from build123d import *

# Parameters (mm, degrees)
SKETCH1_R             = 60.625
SKETCH1_R_2           = 45
BOSS_EXTRUDE1_DEPTH   = 4
SKETCH2_R             = 49
SKETCH2_R_2           = 45
BOSS_EXTRUDE2_DEPTH   = 50.5
SKETCH4_W             = 8
SKETCH4_H             = 40.5
BOSS_EXTRUDE4_DEPTH   = 7
SKETCH4_W_2           = 27
SKETCH4_H_2           = 10
BOSS_EXTRUDE4_2_DEPTH = 7
BOSS_EXTRUDE5_DEPTH   = 4
SKETCH6_R             = 5
CUT_EXTRUDE2_DEPTH    = 52
CUT_EXTRUDE6_DEPTH    = 100.503925853
SKETCH15_R            = 0.5
CUT_EXTRUDE7_DEPTH    = 4.5
SKETCH15_3_R          = 0.5
CUT_EXTRUDE8_DEPTH    = 4.5
BOSS_EXTRUDE6_DEPTH   = 6.75


with BuildPart() as part:
    # Sketch1 → Boss-Extrude1 (new body)
    with BuildSketch(Plane(origin=(0, 0, 0), x_dir=(1, 0, 0), z_dir=(0, 1, 0))):
        with Locations(Location((0, 0, 0), (0, 0, 270))):
            Circle(SKETCH1_R)
        with Locations(Location((0, 0, 0), (0, 0, 270))):
            Circle(SKETCH1_R_2, mode=Mode.SUBTRACT)
    extrude(amount=BOSS_EXTRUDE1_DEPTH)

    # Sketch2 → Boss-Extrude2 (add)
    with BuildSketch(Plane(origin=(0, 4, 0), x_dir=(1, 0, 0), z_dir=(0, 1, 0))):
        with Locations(Location((0, 0, 0), (0, 0, 270))):
            Circle(SKETCH2_R)
        with Locations(Location((0, 0, 0), (0, 0, 270))):
            Circle(SKETCH2_R_2, mode=Mode.SUBTRACT)
    extrude(amount=BOSS_EXTRUDE2_DEPTH)



with BuildPart() as body_2:
    # Sketch4 → Boss-Extrude4 (new, symmetric)
    with BuildSketch(Plane.XY):
        with Locations((10, 20.25)):
            Rectangle(SKETCH4_W, SKETCH4_H)
    extrude(amount=BOSS_EXTRUDE4_DEPTH, both=True)


with BuildPart() as body_3:
    # Sketch4 → Boss-Extrude4 2 (new, symmetric)
    with BuildSketch(Plane.XY):
        with Locations((-30.5, 35.5)):
            Rectangle(SKETCH4_W_2, SKETCH4_H_2)
    extrude(amount=BOSS_EXTRUDE4_2_DEPTH, both=True)

    # Sketch15<3> → Cut-Extrude8 (cut)
    with BuildSketch(Plane(origin=(0, 40.5, 0), x_dir=(1, 0, 0), z_dir=(0, 1, 0))):
        with Locations(Location((-19.5, 0, 0), (0, 0, 270))):
            Circle(SKETCH15_3_R)
        with Locations(Location((8.5, 0, 0), (0, 0, 270))):
            Circle(SKETCH15_3_R)
    extrude(amount=-CUT_EXTRUDE8_DEPTH, mode=Mode.SUBTRACT)


with BuildPart() as part_1:
    add(part.part)

    add(body_2.part)  # Boss-Extrude5 merges body 2
    # Sketch5 → Boss-Extrude5 (add)
    with BuildSketch(Plane(origin=(0, 0, 0.832419338), x_dir=(1, 0, 0), z_dir=(0, -1, 0))):
        with BuildLine():
            Line((0.92268666, 14.579552818), (36.10584122, 30.137929754))
            ThreePointArc((36.10584122, 30.137929754), (47.46850162, -1.287411864), (36.651216878, -32.904630242))
            Line((36.651216878, -32.904630242), (0.92268666, -16.029114558))
            Line((0.92268666, -16.029114558), (0.92268666, 14.579552818))
        make_face()
    extrude(amount=-BOSS_EXTRUDE5_DEPTH)

    # Sketch6 → Cut-Extrude2 (cut)
    with BuildSketch(Plane.XY):
        with Locations(Location((-11.847358964, 24.485616242, 0), (0, 0, 180))):
            Circle(SKETCH6_R)
    extrude(amount=CUT_EXTRUDE2_DEPTH, mode=Mode.SUBTRACT)

    # Sketch11 → Cut-Extrude6 (cut, through all)
    with BuildSketch(Plane(origin=(0, 4, 0), x_dir=(1, 0, 0), z_dir=(0, 1, 0))):
        with BuildLine():
            Line((16.265526008, 12.732401326), (16.265526008, -6.549664017))
            Line((16.265526008, -6.549664017), (5.714961953, -6.549664017))
            Line((5.714961953, -6.549664017), (5.714961953, -11.643039768))
            Line((5.714961953, -11.643039768), (30.818028154, -22.557416377))
            ThreePointArc((30.818028154, -22.557416377), (39.374347706, -1.214976289), (32.152007517, 20.615006655))
            Line((32.152007517, 20.615006655), (16.265526008, 12.732401326))
        make_face()
    extrude(amount=-CUT_EXTRUDE6_DEPTH, mode=Mode.SUBTRACT)

    # Sketch15 → Cut-Extrude7 (cut)
    with BuildSketch(Plane(origin=(0, 40.5, 0), x_dir=(1, 0, 0), z_dir=(0, 1, 0))):
        with Locations((-19.5, 0)):
            Circle(SKETCH15_R)
        with Locations(Location((8.5, 0, 0), (0, 0, 270))):
            Circle(SKETCH15_R)
    extrude(amount=-CUT_EXTRUDE7_DEPTH, mode=Mode.SUBTRACT)


    add(body_3.part)  # Boss-Extrude6 merges body 3
    # Sketch17 → Boss-Extrude6 (add, symmetric)
    with BuildSketch(Plane.XY):
        Polygon((-17, 30.5), (-45, 30.5), (-45, 12.445827276), (-18.590132897, 25.433454532), align=None)
    extrude(amount=BOSS_EXTRUDE6_DEPTH, both=True)


solid = part_1.part
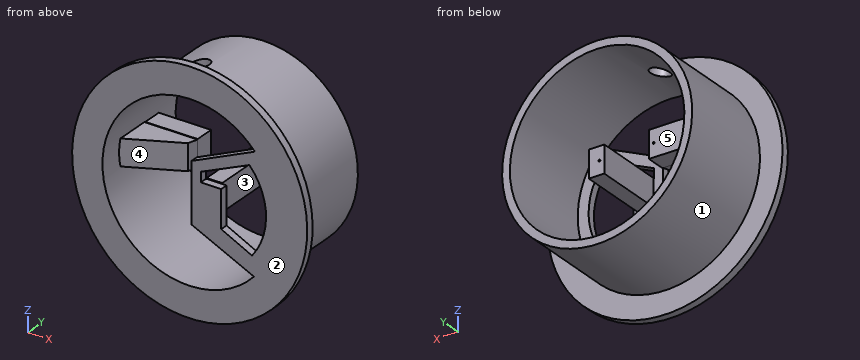
Design review of the part built by this model. Coordinates are the model's own, in mm. Face numbers are marked on the shaded views. A direction names the side the tool comes from. Give positions to 0.01 mm unless a question says otherwise; leave off trailing zeros. Order: outer loops, then holes, each group sorted by start corner. A loop starts at its lowest first (then second) coordinate and runs counter-clockwise, first axis right, second up. Notation, with made-up numbers: (52, 27) - (72, 27) arc R4 cw to (72, 33) - close; hole circle Ø9 at (81.25, -10). An arc over 180 degrees is marked (long way). Write item = value, one per line. Start each with the question number.
Q1. We need section D-D on z = 17.5. State the section outline as (x, y) points, plus the area to 3 significant figures.
Q2. Clearance check with flat-ended pins moving along their axes: pin 1 Ø8 at (x, y) = (-26, 36) entering from -Z; pin 2 Ø12 at (x, y) = (46.5, 6.5) entering from -Z; pin 3 Ø1 at (x, y) = (-44, 19) entering from -Z. State where each tip first meets the part, or that it passes through.
Q3. We need section B-B on x = -5. State the section outline as (y, z) points.
Q4. Mouldability with a two-part tool opening along Z and no side actions: class the marked faces 1, 2 and 3 as released by +Z, released by -Z, zero draft, split by the parting line, or undercut.
Q5. We need section C-C on z = -32. State the section outline as (x, y) points.
Q6. We need section A-A on y = 10.5. State the section outline as (x, z) points, plus the area to 3 significant figures.
Q7. Tool access review of the marked faces 4 and 5: name each direction out of +Z, -Z, +X, -X, +Y, -Y from which nothing blocks a thin tool from reaching the whole face with its end or side.
Q8. To check wall thickness, follow L1, parallel to X at y = 38.85, z = 0; L2, parallel to X at y = 34, z = 0; L3, parallel to X at y = 6, z = -1.5 (3 decimals). State the ranges of each line that lie inside material, in increasing order. Write a range as from..to.
Working result:
q1.outline = (-58.04, 0) - (-41.46, 0) - (-41.46, 54.5) - (-45.77, 54.5) - (-45.77, 4) - (-58.04, 4) - close; (5.64, 0) - (19.19, 0) - (19.19, 4) - (5.64, 4) - close; (34.56, 0) - (58.04, 0) - (58.04, 4) - (45.77, 4) - (45.77, 54.5) - (41.46, 54.5) - (41.46, 4) - (34.56, 4) - close
q1.area = 650 mm²
q2.pin_1 = -43.78
q2.pin_2 = -44.62
q2.pin_3 = -22.56
q3.outline = (0, -60.42) - (4, -60.42) - (4, -48.74) - (54.5, -48.74) - (54.5, -44.72) - (0, -44.72) - close; (0, 44.72) - (54.5, 44.72) - (54.5, 48.74) - (4, 48.74) - (4, 60.42) - (0, 60.42) - close
q4.face_1 = split by the parting line
q4.face_2 = zero draft
q4.face_3 = undercut
q5.outline = (-51.49, 0) - (-31.64, 0) - (-31.64, 54.5) - (-37.11, 54.5) - (-37.11, 4) - (-51.49, 4) - close; (31.64, 0) - (51.49, 0) - (51.49, 4) - (37.11, 4) - (37.11, 54.5) - (31.64, 54.5) - close
q6.outline = circle Ø98 at (0, 0); (6, -7) - (14, -7) - (14, 7) - (6, 7) - close; hole circle Ø90 at (0, 0)
q6.area = 1,290 mm²
q7.face_4 = -Y
q7.face_5 = +Y
q8.L1 = -49..-45, -44..-20, -19..-17, 6..8, 9..14, 45..49
q8.L2 = -49..-45, -44..-17, 6..14, 45..49
q8.L3 = -48.977..-44.975, 6..14, 44.975..48.977
